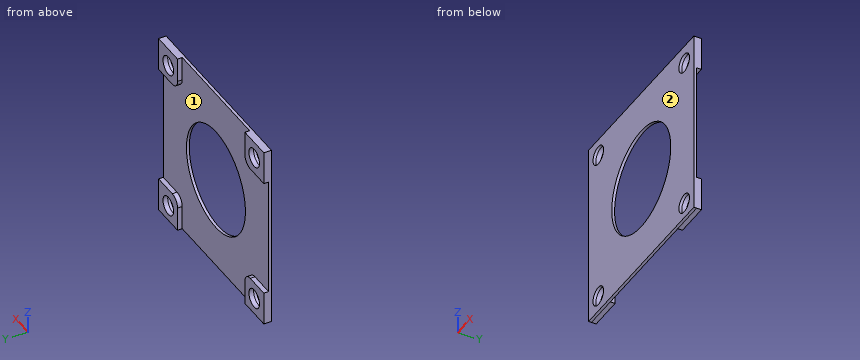
```python
from build123d import *

# Parameters (mm, degrees)
F0_R     = 5
F0_R_2   = 28
F1_DEPTH = 1.5
F2_DEPTH = 2.5


with BuildPart() as f1:
    # F0 (on Front) → F1 (new body)
    with BuildSketch(Plane.XZ):
        with BuildLine():
            Line((-32, 50), (-50, 50))
            Line((-50, 50), (-50, 32))
            Line((-50, 32), (-37, 32))
            ThreePointArc((-37, 32), (-33.464466, 33.464466), (-32, 37))
            Line((-32, 37), (-32, 50))
        make_face()
        with Locations((-40.800001, 40.95)):
            Circle(F0_R, mode=Mode.SUBTRACT)
        with BuildLine():
            Line((50, 50), (32, 50))
            Line((32, 50), (32, 37))
            ThreePointArc((32, 37), (33.464466, 33.464466), (37, 32))
            Line((37, 32), (50, 32))
            Line((50, 32), (50, 50))
        make_face()
        with Locations((40.800005, 40.350001)):
            Circle(F0_R, mode=Mode.SUBTRACT)
        with BuildLine():
            Line((50, -50), (50, -32))
            Line((50, -32), (37, -32))
            ThreePointArc((37, -32), (33.464466, -33.464466), (32, -37))
            Line((32, -37), (32, -50))
            Line((32, -50), (50, -50))
        make_face()
        with Locations((40.800005, -41.550003)):
            Circle(F0_R, mode=Mode.SUBTRACT)
        with BuildLine():
            Line((-37, -32), (-50, -32))
            Line((-50, -32), (-50, -50))
            Line((-50, -50), (-32, -50))
            Line((-32, -50), (-32, -37))
            ThreePointArc((-32, -37), (-33.464466, -33.464466), (-37, -32))
        make_face()
        with Locations((-40.800001, -41.250005)):
            Circle(F0_R, mode=Mode.SUBTRACT)
        with BuildLine():
            Line((32, 50), (-32, 50))
            Line((-32, 50), (-32, 37))
            ThreePointArc((-32, 37), (-33.464466, 33.464466), (-37, 32))
            Line((-37, 32), (-50, 32))
            Line((-50, 32), (-50, -32))
            Line((-50, -32), (-37, -32))
            ThreePointArc((-37, -32), (-33.464466, -33.464466), (-32, -37))
            Line((-32, -37), (-32, -50))
            Line((-32, -50), (32, -50))
            Line((32, -50), (32, -37))
            ThreePointArc((32, -37), (33.464466, -33.464466), (37, -32))
            Line((37, -32), (50, -32))
            Line((50, -32), (50, 32))
            Line((50, 32), (37, 32))
            ThreePointArc((37, 32), (33.464466, 33.464466), (32, 37))
            Line((32, 37), (32, 50))
        make_face()
        Circle(F0_R_2, mode=Mode.SUBTRACT)
    extrude(amount=F1_DEPTH)

    # F0 (on Front) → F2 (join)
    with BuildSketch(Plane.XZ):
        with BuildLine():
            Line((-32, 50), (-50, 50))
            Line((-50, 50), (-50, 32))
            Line((-50, 32), (-37, 32))
            ThreePointArc((-37, 32), (-33.464466, 33.464466), (-32, 37))
            Line((-32, 37), (-32, 50))
        make_face()
        with Locations((-40.800001, 40.95)):
            Circle(F0_R, mode=Mode.SUBTRACT)
        with BuildLine():
            Line((50, 50), (32, 50))
            Line((32, 50), (32, 37))
            ThreePointArc((32, 37), (33.464466, 33.464466), (37, 32))
            Line((37, 32), (50, 32))
            Line((50, 32), (50, 50))
        make_face()
        with Locations((40.800005, 40.350001)):
            Circle(F0_R, mode=Mode.SUBTRACT)
        with BuildLine():
            Line((-37, -32), (-50, -32))
            Line((-50, -32), (-50, -50))
            Line((-50, -50), (-32, -50))
            Line((-32, -50), (-32, -37))
            ThreePointArc((-32, -37), (-33.464466, -33.464466), (-37, -32))
        make_face()
        with Locations((-40.800001, -41.250005)):
            Circle(F0_R, mode=Mode.SUBTRACT)
        with BuildLine():
            Line((50, -50), (50, -32))
            Line((50, -32), (37, -32))
            ThreePointArc((37, -32), (33.464466, -33.464466), (32, -37))
            Line((32, -37), (32, -50))
            Line((32, -50), (50, -50))
        make_face()
        with Locations((40.800005, -41.550003)):
            Circle(F0_R, mode=Mode.SUBTRACT)
    extrude(amount=-F2_DEPTH)


solid = f1.part
```
Check sheet for the modelled part. Datum: model origin and axes. Units: mm. Face numbers are marked on the shaded views. Coordinates: 2 decimals unless noted, no trailing zeros. Loops run counter-clockwise (first coordinate to the right, second up) from the corner with the lowest first, then second, coordinate; pieces in that order, holes last.
1) Material ranges on probe 1 along Z at (x, y) = (-1, -0.8); probe 2 along X at (y, z) = (-0.15, 41); probe 3 along X at (y, z) = (0.8, 38), recorded low to high.
2) Sectioned sample at C-C (z = 0). Record the boundary of the cut face in (x, y).
3) Gauge pin test, flat end, axial feed: pin 1 (2 mm diameter, centred on x = -36, z = -10, fed in from +Y). Record the tip position at first contact, or that the pin passes through.
4) Sectioned sample at B-B (x = 0). Record the boundary of the cut face in (y, z).
5) Sectioned sample at A-A (y = 1.05). Record the boundary of the cut face in (x, z).
6) Release check for a two-part mould opening along Z. For the marked faces 1 and 2 record: released by +Z, released by -Z, zero draft, split by the parting line, or undercut.
Check sheet entries:
1. probe 1: z = -50 to -27.98, 27.98 to 50
1. probe 2: x = -50 to -45.8, -35.8 to 35.84, 45.76 to 50
1. probe 3: x = -50 to -44.84, -36.76 to -32, 32 to 36.39, 45.21 to 50
2. outline: (-50, -1.5) - (-28, -1.5) - (-28, 0) - (-50, 0) - close; (28, -1.5) - (50, -1.5) - (50, 0) - (28, 0) - close
3. pin 1: stops at y = 0
4. outline: (-1.5, -50) - (0, -50) - (0, -28) - (-1.5, -28) - close; (-1.5, 28) - (0, 28) - (0, 50) - (-1.5, 50) - close
5. outline: (-50, -50) - (-32, -50) - (-32, -37) arc R5 ccw to (-37, -32) - (-50, -32) - close; (-50, 32) - (-37, 32) arc R5 ccw to (-32, 37) - (-32, 50) - (-50, 50) - close; (32, -50) - (50, -50) - (50, -32) - (37, -32) arc R5 ccw to (32, -37) - close; (32, 37) arc R5 ccw to (37, 32) - (50, 32) - (50, 50) - (32, 50) - close; hole circle Ø10 at (-40.8, -41.25); hole circle Ø10 at (-40.8, 40.95); hole circle Ø10 at (40.8, -41.55); hole circle Ø10 at (40.8, 40.35)
6. face 1: undercut
6. face 2: zero draft
